Verification items for the finished model (mm, model axes). Face numbers are marked on the shaded views. Coordinates: 2 decimals unless noted, no trailing zeros. Order: outer loops, then holes, each group sorted by start corner. A loop starts at its lowest first (then second) coordinate and runs counter-clockwise, first axis right, second up. Notation, with made-up numbers: M -4,36.5 L 11,36.5 A29 cw 11,70.5 Z; hole C 40.5,39.5 d4. An arc over 180 degrees is marked long. Return JSON: item names as keys, results as strings. Group by question number.
1. Mould release check, pull along X, two halves, no side actions. Record for the marked faces 1 and 2: +X half, -X half, draft (parallel to the pull), parting line (faces both ways), or undercut.
2. Section check B-B, the plane y = 0.95. Record the cut outline in (x, z), plus the area to 3 significant figures.
3. Gauge pin test, flat ends, axial feed: pin 1 (1 mm diameter, centred on x = -1.5, y = 2, fed in from -Z); pin 2 (1 mm diameter, centred on y = 2.5, z = 11, fed in from +X). Record the tip position at first contact, or that the pin passes through.
4. Material ranges on line 1 along Z through (x, y) = (0.25, 1.9) (3 decimals); line 2 along Z through (x, y) = (-1.5, 2.55); line 3 along X through (y, z) = (1.35, 10), recorded low to high.
5. Section check A-A, the plane z = 0. Record the cut outline in (x, y).
```python
from build123d import *

# Parameters (mm, degrees)
SKETCH1_R           = 15
BOSS_EXTRUDE1_DEPTH = 3
SKETCH2_R           = 1.09
CUT_EXTRUDE1_DEPTH  = 3
CIRPATTERN1_COUNT   = 4
FILLET1_R           = 0.5
SKETCH5_R           = 6.25
CUT_EXTRUDE2_DEPTH  = 25


with BuildPart() as part:
    # Sketch1 → Boss-Extrude1 (new body)
    with BuildSketch(Plane(origin=(0, 0, 0), x_dir=(1, 0, 0), z_dir=(0, 1, 0))):
        with Locations(Location((0, 0, 0), (0, 0, 270))):
            Circle(SKETCH1_R)
    extrude(amount=BOSS_EXTRUDE1_DEPTH)

    # Sketch2 → Cut-Extrude1 (cut)
    with BuildSketch(Plane(origin=(0, 3, 0), x_dir=(1, 0, 0), z_dir=(0, 1, 0))):
        with Locations(Location((0, 10, 0), (0, 0, 270))):
            Circle(SKETCH2_R)
    cut_extrude1 = extrude(amount=-CUT_EXTRUDE1_DEPTH, mode=Mode.SUBTRACT)

    # CirPattern1: Cut-Extrude1 ×4 about axis
    cirpattern1_axis = Axis((0, 0, 0), (0, 1, 0))
    for i in range(1, CIRPATTERN1_COUNT):
        add(cut_extrude1.rotate(cirpattern1_axis, i * 360 / CIRPATTERN1_COUNT), mode=Mode.SUBTRACT)

    # Fillet1
    fillet1_edges = [part.edges().sort_by_distance(p)[0] for p in [
        (0, 0, -15),
        (0, 3, -15),
    ]]
    fillet(fillet1_edges, radius=FILLET1_R)

    # Sketch5 → Cut-Extrude2 (cut, symmetric)
    with BuildSketch(Plane(origin=(0, 3, 0), x_dir=(1, 0, 0), z_dir=(0, 1, 0))):
        with Locations(Location((0, 0, 0), (0, 0, 270))):
            Circle(SKETCH5_R)
    extrude(amount=CUT_EXTRUDE2_DEPTH, both=True, mode=Mode.SUBTRACT)


solid = part.part
```
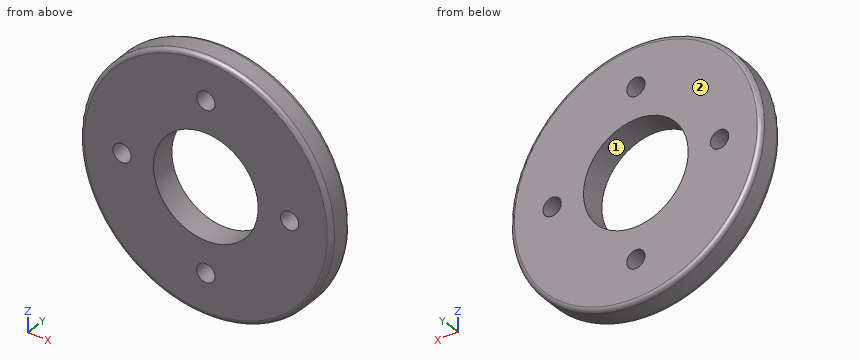
Answers follow:
{
 "1": {"face 1": "undercut", "face 2": "draft"},
 "2": {"outline": "C 0,0 d30; hole C -10,0 d2.18; hole C 0,0 d12.5; hole C 0,-10 d2.18; hole C 0,10 d2.18; hole C 10,0 d2.18", "area": "569 mm^2"},
 "3": {"pin 1": "z = -14.97", "pin 2": "x = 10.71"},
 "4": {"line 1": "-14.998 to -11.061, -8.939 to -6.245, 6.245 to 8.939, 11.061 to 14.998", "line 2": "-14.92 to -6.07, 6.07 to 14.92", "line 3": "-11.18 to -1.09, 1.09 to 11.18"},
 "5": {"outline": "M -15,0.5 A0.5 ccw -14.5,0 L -11.09,0 L -11.09,3 L -14.5,3 A0.5 ccw -15,2.5 Z; M -8.91,0 L -6.25,0 L -6.25,3 L -8.91,3 Z; M 6.25,0 L 8.91,0 L 8.91,3 L 6.25,3 Z; M 11.09,0 L 14.5,0 A0.5 ccw 15,0.5 L 15,2.5 A0.5 ccw 14.5,3 L 11.09,3 Z"}
}
